Read the model definition and answer for the solid it produces. Units are mm, in the model's axes. Face numbers are marked on the shaded views. A direction names the side the tool comes from. Coordinates: 2 decimals unless noted, no trailing zeros. Order: outer loops, then holes, each group sorted by start corner. A loop starts at its lowest first (then second) coordinate and runs counter-clockwise, first axis right, second up. Notation, with made-up numbers: (-29, -38) - (19, -38) arc R20 cw to (19, -34) - close; hole circle Ø4 at (53, 32). An arc over 180 degrees is marked (long way). Write item = value, one per line.
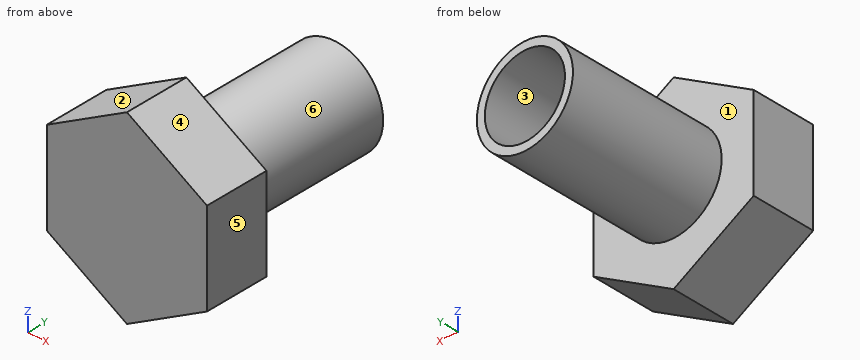
from build123d import *

# Parameters (mm, degrees)
SKETCH1_R           = 3
SKETCH1_R_2         = 2.5
BOSS_EXTRUDE1_DEPTH = 10
BOSS_EXTRUDE2_DEPTH = 4


with BuildPart() as part:
    # Sketch1 → Boss-Extrude1 (new body)
    with BuildSketch(Plane(origin=(0, 0, 0), x_dir=(1, 0, 0), z_dir=(0, 1, 0))):
        Circle(SKETCH1_R)
        Circle(SKETCH1_R_2, mode=Mode.SUBTRACT)
    extrude(amount=BOSS_EXTRUDE1_DEPTH)

    # Sketch2 → Boss-Extrude2 (add)
    with BuildSketch(Plane.XZ):
        Polygon((0, 5.773502692), (-5, 2.886751346), (-5, -2.886751346), (0, -5.773502692), (5, -2.886751346), (5, 2.886751346), align=None)
    extrude(amount=BOSS_EXTRUDE2_DEPTH)


solid = part.part
1) Straight lines are drawn through the part: line 1 along Z through (x, y) = (0, 7); line 2 along Y through (x, z) = (-1, 0.75). For each, find the intervals that lie inside material, in ascending order. Write a range as from..to.
Returned:
line_1 = -3..-2.5, 2.5..3
line_2 = -4..0
2) The part is cut by section D-D (x = -4). Determine the outline of the cut face in (y, z), and give its area (3 significant figures).
Returned:
outline = (-4, -3.46) - (0, -3.46) - (0, 3.46) - (-4, 3.46) - close
area = 27.7 mm^2
3) The part is cut by section B-B (x = -0.5). Determine the outline of the cut face in (y, z).
Returned:
outline = (-4, -5.48) - (0, -5.48) - (0, -2.96) - (10, -2.96) - (10, -2.45) - (0, -2.45) - (0, 2.45) - (10, 2.45) - (10, 2.96) - (0, 2.96) - (0, 5.48) - (-4, 5.48) - close
4) Flat-ended cylindrical pins translate along their axes: pin 1 Ø1 at (y, z) = (5.5, -1.5) entering from -X; pin 2 Ø1.5 at (x, z) = (-1, -0.5) entering from +Y. Find the tip coordinate at first contact, or state that the pin passes through.
Returned:
pin_1 = -2.83
pin_2 = 0
5) The part is cut by section A-A (y = -2.5). Determine the outline of the cut face in (x, z).
Returned:
outline = (-5, -2.89) - (0, -5.77) - (5, -2.89) - (5, 2.89) - (0, 5.77) - (-5, 2.89) - close
6) For the marked faces 1 and 2, determine the directions among +Z, -Z, +X, -X, +Y, -Y from which every point of the face is accessible in a straight line to the end or side of a thin tool.
Returned:
face_1 = +Y
face_2 = +Z, -X, +Y, -Y
7) Determine the mould class of the marked faces 3, 4, 5 and 6 for opening direction Z: pulls with the +Z half, pulls with the -Z half, needs draft (parallel to the pull), parting line crosses it, or undercut.
Returned:
face_3 = undercut
face_4 = pulls with the +Z half
face_5 = needs draft
face_6 = parting line crosses it
8) The part is cut by section C-C (z = -4.5). Determine the outline of the cut face in (x, y).
Returned:
outline = (-2.21, -4) - (2.21, -4) - (2.21, 0) - (-2.21, 0) - close
